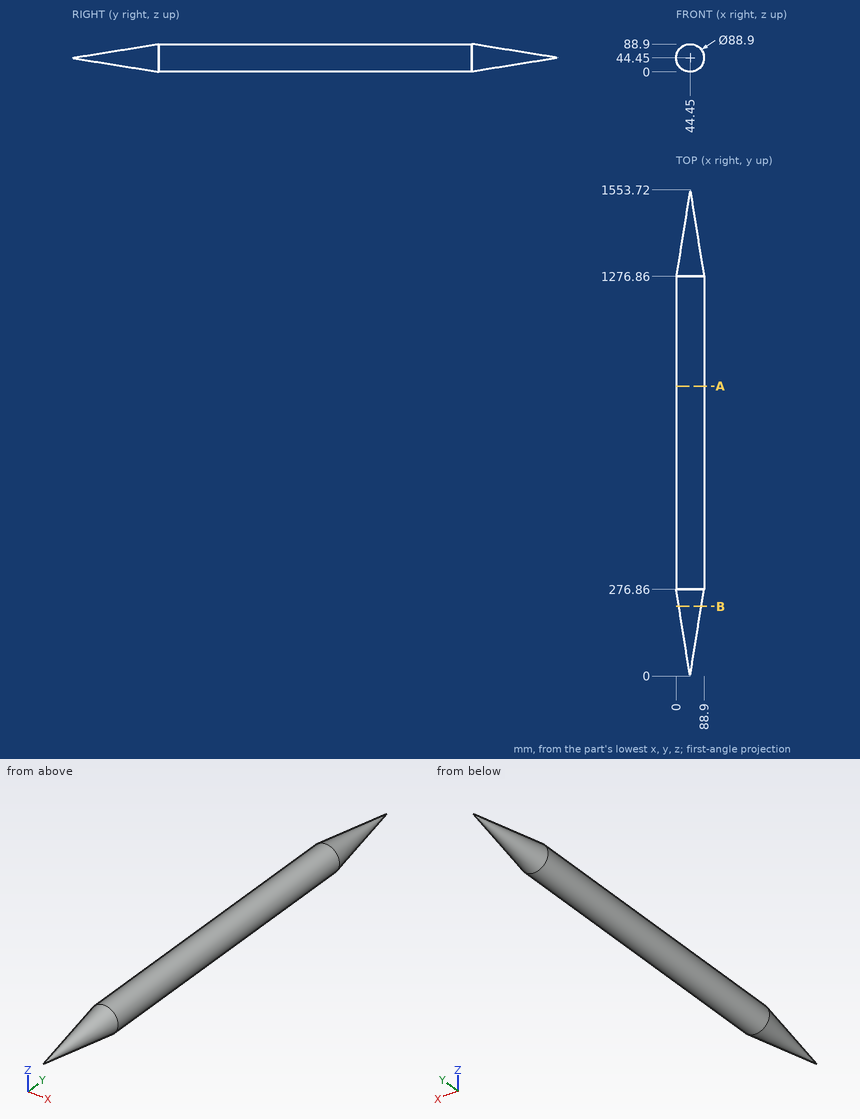
Here's the drawing with two shaded views (mm, measured from the low corner). I have some questions. Give positions to 0.01 mm unless a question says otherwise; leave off trailing zeros. Loops run counter-clockwise (first coordinate to the right, second up) from the corner with the lowest first, then second, coordinate; pieces in that order, holes last. Notation, with made-up numbers: M 84,38 L 112,38 A17 ccw 112,57 Z; hole C 19.25,17.25 d10. An arc over 180 degrees is marked long. Use one line per item in the form item = value. Start each with the question number.
(1) I want a section at A-A, the plane y = 926.5. Write out the boundary of the cut face in (x, z).
(2) I want a section at B-B, the plane y = 222.5. Write out the boundary of the cut face in (x, z).
(3) Please list where these lines run through material, in increasing order: line 1 (Z direction, x = 45.5, y = 311); line 2 (Z direction, x = 39, y = 1417.5); line 3 (X direction, y = 1456, z = 44).
(4) I'm going to push flat-ended pins straight in: P1, Ø3, axis at y = 822, z = 73, coming from the +X side; P2, Ø6, axis at y = 609, z = 43.5, coming from the -X side; P3, Ø1.5, axis at x = 61, y = 1326, coming from the -Z side; P4, Ø1.5, axis at x = 43, y = 466, coming from the +Z side. Where does each tip first touch, or does it pass through?
Worked out:
q1.outline = C 44.45,44.45 d88.9
q2.outline = C 44.45,44.45 d71.44
q3.line_1 = 0.01 to 88.89
q3.line_2 = 23.27 to 65.63
q3.line_3 = 28.77 to 60.13
q4.P1 = 79.72
q4.P2 = 0
q4.P3 = 11.46
q4.P4 = 88.89
